Autodesk Inventor part; units mm, degrees
ref_plane "YZ Plane" through (0, 0, 0) normal (1, 0, 0) x (0, 1, 0)
ref_plane "XZ Plane" through (0, 0, 0) normal (0, 1, 0) x (-1, 0, 0)
ref_plane "XY Plane" through (0, 0, 0) normal (0, 0, 1) x (1, 0, 0)
sketch "Sketch1" plane through (0, 0, 0) normal (0, 0, 1) x (1, 0, 0)
  circle A0 centre (-18.1795, -61.2779) radius 2.413
  circle A1 centre (102.2419, -61.2779) radius 2.413
  line L0 (-23.2595, -45.4029) -> (-23.2595, -64.9896) construction
  line L1 (107.3219, -48.5779) -> (107.3219, -70.0812) construction
  line L2 (116.8469, -45.4029) -> (-32.7845, -45.4029)
  line L3 (120.0219, -48.5779) -> (120.0219, -112.0779)
  line L4 (116.8469, -115.2529) -> (-32.7845, -115.2529)
  line L5 (-35.9595, -112.0779) -> (-35.9595, -48.5779)
  arc A2 (-32.7845, -45.4029) -> (-35.9595, -48.5779) centre (-32.7845, -48.5779) ccw
  arc A3 (-35.9595, -112.0779) -> (-32.7845, -115.2529) centre (-32.7845, -112.0779) ccw
  arc A4 (116.8469, -115.2529) -> (120.0219, -112.0779) centre (116.8469, -112.0779) ccw
  arc A5 (120.0219, -48.5779) -> (116.8469, -45.4029) centre (116.8469, -48.5779) ccw
  line L6 (-29.6095, -50.4829) -> (-23.2595, -50.4829)
  line L7 (-23.2595, -50.4829) -> (-23.2595, -65.7229)
  line L8 (-23.2595, -65.7229) -> (-29.6095, -65.7229)
  line L9 (-29.6095, -65.7229) -> (-29.6095, -50.4829)
  line L10 (-29.6095, -72.0729) -> (-23.2595, -72.0729)
  line L11 (-23.2595, -72.0729) -> (-23.2595, -87.3129)
  line L12 (-23.2595, -87.3129) -> (-29.6095, -87.3129)
  line L13 (-29.6095, -87.3129) -> (-29.6095, -72.0729)
  line L14 (-29.6095, -93.6629) -> (-23.2595, -93.6629)
  line L15 (-23.2595, -93.6629) -> (-23.2595, -108.9029)
  line L16 (-23.2595, -108.9029) -> (-29.6095, -108.9029)
  line L17 (-29.6095, -108.9029) -> (-29.6095, -93.6629)
  line L18 (42.0312, -45.4029) -> (42.0312, -115.2529) construction
  line L19 (113.6719, -50.4829) -> (107.3219, -50.4829)
  line L20 (107.3219, -50.4829) -> (107.3219, -65.7229)
  line L21 (107.3219, -65.7229) -> (113.6719, -65.7229)
  line L22 (113.6719, -65.7229) -> (113.6719, -50.4829)
  line L23 (113.6719, -72.0729) -> (107.3219, -72.0729)
  line L24 (107.3219, -72.0729) -> (107.3219, -87.3129)
  line L25 (107.3219, -87.3129) -> (113.6719, -87.3129)
  line L26 (113.6719, -87.3129) -> (113.6719, -72.0729)
  line L27 (113.6719, -93.6629) -> (107.3219, -93.6629)
  line L28 (107.3219, -93.6629) -> (107.3219, -108.9029)
  line L29 (107.3219, -108.9029) -> (113.6719, -108.9029)
  line L30 (113.6719, -108.9029) -> (113.6719, -93.6629)
  line L31 (-16.9095, -102.5529) -> (-1.6695, -102.5529)
  line L32 (-1.6695, -102.5529) -> (-1.6695, -108.9029)
  line L33 (-1.6695, -108.9029) -> (-16.9095, -108.9029)
  line L34 (-16.9095, -108.9029) -> (-16.9095, -102.5529)
  line L35 (13.5705, -102.5529) -> (28.8105, -102.5529)
  line L36 (28.8105, -102.5529) -> (28.8105, -108.9029)
  line L37 (28.8105, -108.9029) -> (13.5705, -108.9029)
  line L38 (13.5705, -108.9029) -> (13.5705, -102.5529)
  line L39 (100.9719, -102.5529) -> (85.7319, -102.5529)
  line L40 (85.7319, -102.5529) -> (85.7319, -108.9029)
  line L41 (85.7319, -108.9029) -> (100.9719, -108.9029)
  line L42 (100.9719, -108.9029) -> (100.9719, -102.5529)
  line L43 (70.4919, -102.5529) -> (55.2519, -102.5529)
  line L44 (55.2519, -102.5529) -> (55.2519, -108.9029)
  line L45 (55.2519, -108.9029) -> (70.4919, -108.9029)
  line L46 (70.4919, -108.9029) -> (70.4919, -102.5529)
  line L47 (-10.5595, -86.0529) -> (2.4405, -86.0529)
  line L48 (2.4405, -86.0529) -> (2.4405, -97.5529)
  line L49 (2.4405, -97.5529) -> (-10.5595, -97.5529)
  line L50 (-10.5595, -97.5529) -> (-10.5595, -86.0529)
  point P0 (0, 0)
  point P1 (-35.9595, -45.4029)
  point P2 (-35.9595, -115.2529)
  point P3 (107.3219, -64.9896)
  dimension "d3" = 4.826
  dimension "d4" = 4.826
  dimension "d7" = 120.4214
  dimension "d8" = 5.08
  dimension "d9" = 5.08
  dimension "d18" = 15.875
  dimension "d19" = 15.875
  dimension "d20" = 90
  dimension "d21" = 12.7
  dimension "d22" = 155.9814
  dimension "d23" = 69.85
  dimension "d24" = 3.175
  dimension "d25" = 6.35
  dimension "d26" = 6.35
  dimension "d27" = 15.24
  dimension "d28" = 15.24
  dimension "d29" = 15.24
  dimension "d30" = 6.35
  dimension "d31" = 6.35
  dimension "d32" = 6.35
  dimension "d37" = 15.24
  dimension "d38" = 15.24
  dimension "d40" = 6.35
  dimension "d41" = 15.24
  dimension "d50" = 6.35
  dimension "d53" = 11.5
  dimension "d54" = 13
  dimension "d55" = 5
  dimension "d56" = 12.7
extrude "Extrusion6" add sketch "Sketch1" along normal blind 6.35
equation "\"d4\" = d3"
equation "\"d19\" = d18"
equation "\"d22\" = 2 * d21 + d7 + d9 + d8"
equation "\"d28\" = d27"
equation "\"d29\" = d27"
equation "\"d31\" = d30"
equation "\"d32\" = d30"
equation "\"d37\" = d27"
equation "\"d38\" = d27"
equation "\"d40\" = d30"
properties part number "Tester Cheek PE" material "UHMW, Black"
Geometry: final body of the model. Coordinates: model frame, mm. A direction names the side the tool comes from. Round coordinates to 2 decimals unless told otherwise and drop trailing zeros. Order: outer loops, then holes, each group sorted by start corner. A loop starts at its lowest first (then second) coordinate and runs counter-clockwise, first axis right, second up. Notation, with made-up numbers: (-38, -21) -> (14, -21) arc R14 ccw to (14, -2) -> close; hole circle Ø8 at (-20, 84.25). An arc over 180 degrees is marked (long way). Put each result on its own line as item: value. Start each with the question number.
Q1. Pull-direction query (X, two-part tool) for faces 1 (the flat face through (41, -80, 0)), 2 (the flat face through (-23.26, -80, 3)), 3 (the cylindrical face through (-35, -114.35, 3.13)); classes: +X half, -X half, draft (parallel to the pull), parting line (faces both ways), or undercut.
Q2. Section B-B on x = -8.5. Return the cut outline in (y, z), and give its area (3 significant figures).
Q3. Line query: probe 1 along X at (y, z) = (-82.5, 3.25); probe 2 along Y at (x, z) = (110, 2.5); probe 3 along Y at (x, z) = (-4.5, 2). Output: solid intervals per line, ascending.
Q4. Section A-A on y = -74. Return the cut outline in (x, z), and give its area (3 significant figures).
Q5. Section D-D on x = 20. Return the cut outline in (y, z).
Q6. Section C-C on y = -105. Return the cut outline in (x, z).
Q7. Reachability of faces 4 (the flat face through (43, -115.253, 3)), 5 (the flat face through (21, -108.903, 3)) from +Z, -Z, +X, -X, +Y, -Y: full face, straight path, thin tool, end or side. Return the list, or none.
Ans:
1. face 1: draft
1. face 2: undercut
1. face 3: -X half
2. outline: (-115.25, 0) -> (-108.9, 0) -> (-108.9, 6.35) -> (-115.25, 6.35) -> close; (-102.55, 0) -> (-97.55, 0) -> (-97.55, 6.35) -> (-102.55, 6.35) -> close; (-86.05, 0) -> (-45.4, 0) -> (-45.4, 6.35) -> (-86.05, 6.35) -> close
2. area: 330 mm2
3. probe 1: x = -35.96 to -29.61, -23.26 to 107.32, 113.67 to 120.02
3. probe 2: y = -115.25 to -108.9, -93.66 to -87.31, -72.07 to -65.72, -50.48 to -45.4
3. probe 3: y = -115.25 to -108.9, -102.55 to -97.55, -86.05 to -45.4
4. outline: (-35.96, 0) -> (-29.61, 0) -> (-29.61, 6.35) -> (-35.96, 6.35) -> close; (-23.26, 0) -> (107.32, 0) -> (107.32, 6.35) -> (-23.26, 6.35) -> close; (113.67, 0) -> (120.02, 0) -> (120.02, 6.35) -> (113.67, 6.35) -> close
4. area: 910 mm2
5. outline: (-115.25, 0) -> (-108.9, 0) -> (-108.9, 6.35) -> (-115.25, 6.35) -> close; (-102.55, 0) -> (-45.4, 0) -> (-45.4, 6.35) -> (-102.55, 6.35) -> close
6. outline: (-35.96, 0) -> (-29.61, 0) -> (-29.61, 6.35) -> (-35.96, 6.35) -> close; (-23.26, 0) -> (-16.91, 0) -> (-16.91, 6.35) -> (-23.26, 6.35) -> close; (-1.67, 0) -> (13.57, 0) -> (13.57, 6.35) -> (-1.67, 6.35) -> close; (28.81, 0) -> (55.25, 0) -> (55.25, 6.35) -> (28.81, 6.35) -> close; (70.49, 0) -> (85.73, 0) -> (85.73, 6.35) -> (70.49, 6.35) -> close; (100.97, 0) -> (107.32, 0) -> (107.32, 6.35) -> (100.97, 6.35) -> close; (113.67, 0) -> (120.02, 0) -> (120.02, 6.35) -> (113.67, 6.35) -> close
7. face 4: +Z, -Z, +X, -X, -Y
7. face 5: +Z, -Z
